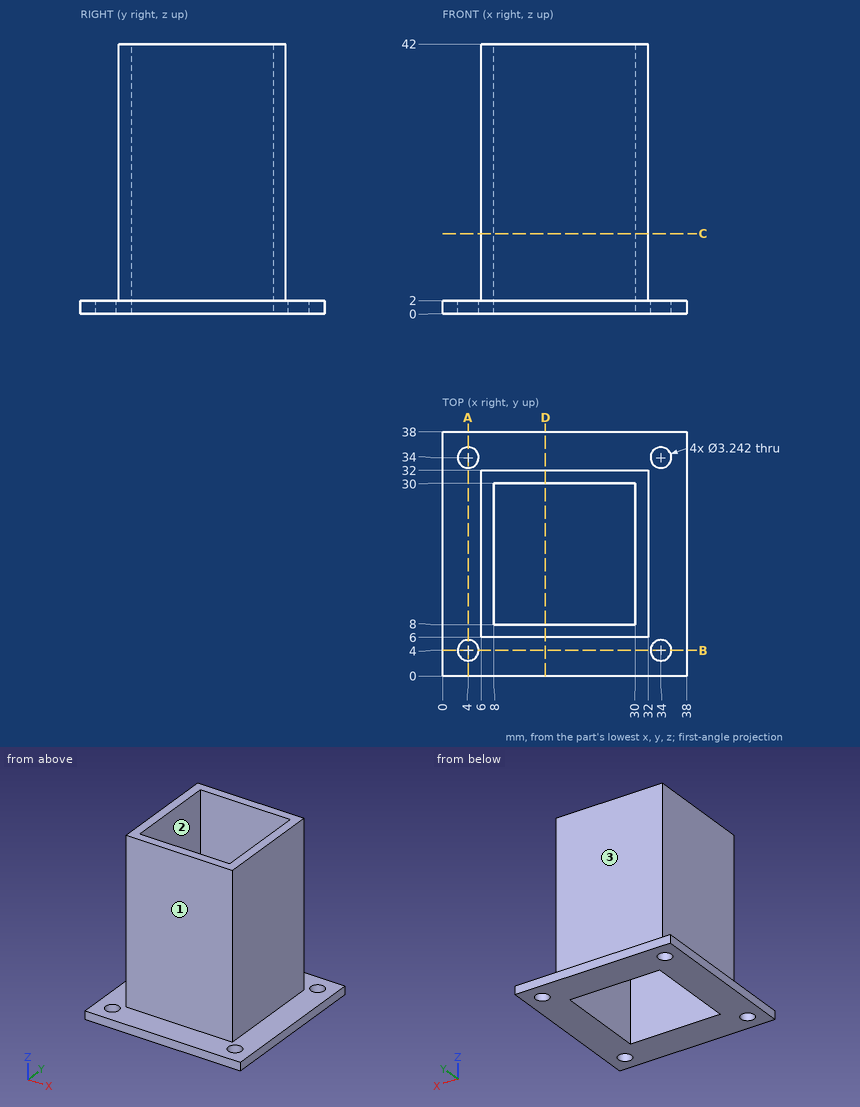
Study the drawing (mm; zero at the part's minimum x, y, z) and answer. A direction names the side the tool comes from. Give positions to 0.01 mm unless a question says otherwise; leave off trailing zeros. Order: outer loops, then holes, each group sorted by start corner. A loop starts at its lowest first (then second) coordinate and runs counter-clockwise, first axis right, second up. Notation, with made-up numbers: M -29.75,-15.5 L 4.25,-15.5 A32 ccw 4.25,14.5 Z; hole C 88,7 d2. An arc over 180 degrees is marked long. Put each result on its own line as item: value. Start each with the question number.
Item 1: Which of the six approach directions +Z, -Z, +X, -X, +Y, -Y give full straight-line access (tool end or side, diameter ignored) to the marked faces 1, 2 and 3?
Item 2: The part is cut by section A-A, the plane x = 4. Determine the outline of the cut face in (y, z).
Item 3: Find the intervals of material crossed by line 1 along Y through (x, z) = (4, 1.3); line 2 along Y through (x, z) = (15, 26.5), in increasing order.
Item 4: The part is cut by section D-D, the plane x = 16. Determine the outline of the cut face in (y, z), and give its area (3 significant figures).
Item 5: Flat-ended cylindrical pins translate along their axes: P1, Ø1, axis at x = 4.5, y = 34, coming from the +Z side; P2, Ø21, axis at y = 16, z = 28, coming from the +X side; P3, Ø12, axis at y = 27, z = 19.5, coming from the -X side; P4, Ø21, axis at x = 18, z = 21.5, coming from the +Y side. Find the tip coordinate at first contact, or state that the pin passes through.
Item 6: The part is cut by section C-C, the plane z = 12.5. Determine the outline of the cut face in (x, y).
Answer key:
1. face 1: +Z, +X, -X, -Y
1. face 2: +Z, -Z
1. face 3: +Z, +X, -X, +Y
2. outline: M 0,0 L 2.38,0 L 2.38,2 L 0,2 Z; M 5.62,0 L 32.38,0 L 32.38,2 L 5.62,2 Z; M 35.62,0 L 38,0 L 38,2 L 35.62,2 Z
3. line 1: y = 0 to 2.38, 5.62 to 32.38, 35.62 to 38
3. line 2: y = 6 to 8, 30 to 32
4. outline: M 0,0 L 8,0 L 8,42 L 6,42 L 6,2 L 0,2 Z; M 30,0 L 38,0 L 38,2 L 32,2 L 32,42 L 30,42 Z
4. area: 192 mm²
5. P1: passes through
5. P2: stops at x = 32
5. P3: stops at x = 6
5. P4: stops at y = 32
6. outline: M 6,6 L 32,6 L 32,32 L 6,32 Z; hole M 8,8 L 30,8 L 30,30 L 8,30 Z
